Source: CAD feature listing. Evaluate the final solid. Frame: model axes, mm. Coordinates: 2 decimals unless noted, no trailing zeros. Order: outer loops, then holes, each group sorted by start corner. A loop starts at its lowest first (then second) coordinate and runs counter-clockwise, first axis right, second up.
```python
from build123d import *

# Parameters (mm, degrees)
EXTRUDE_1_DEPTH     = 2
SKETCH_2_R          = 3
SKETCH_2_R_2        = 0.8
CUT_EXTRUDE_1_DEPTH = 2
FILLET_1_R          = 2
FILLET_3_R          = 16


with BuildPart() as part:
    # Эскиз1 → Бобышка-Вытянуть1 (new body)
    with BuildSketch(Plane(origin=(0, 0, 0), x_dir=(0, 0, -1), z_dir=(1, 0, 0))):
        Polygon((-17.95, 0), (-3.95, 8), (3.95, 8), (17.95, 0), (17.95, -10), (-17.95, -10), align=None)
    extrude(amount=EXTRUDE_1_DEPTH)

    # Эскиз2 → Вырез-Вытянуть1 (cut)
    with BuildSketch(Plane(origin=(2, 0, 0), x_dir=(0, 0, -1), z_dir=(1, 0, 0))):
        with Locations((6.34428877, -4)):
            Circle(SKETCH_2_R)
        with Locations((1.84428877, -4)):
            Circle(SKETCH_2_R_2)
        with Locations((10.84428877, -4)):
            Circle(SKETCH_2_R_2)
    extrude(amount=-CUT_EXTRUDE_1_DEPTH, mode=Mode.SUBTRACT)

    # Скругление1
    fillet_1_edges = [part.edges().sort_by_distance(p)[0] for p in [
        (1, 0, 17.95),
        (1, 0, -17.95),
    ]]
    fillet(fillet_1_edges, radius=FILLET_1_R)

    # Скругление3
    # the kernel refuses this fillet: 16 mm, written as the material it takes off along each edge
    with BuildSketch(Plane(origin=(-10.622577483, 8, -3.95), x_dir=(0, 0, 1), z_dir=(1, 0, 0)), Plane(origin=(-10.622577483, 8, 3.95), x_dir=(0, -0.496138938356834, 0.868243142124459), z_dir=(1, 0, 0))) as fillet_3_piece_1:
        with BuildLine():
            CenterArc((FILLET_3_R * 0.265564437075, FILLET_3_R), FILLET_3_R, 240.255118703, 29.744881297)
            Line((-FILLET_3_R * 0.230574501282, FILLET_3_R * 0.131756857876), (0, 0))
            Line((0, 0), (FILLET_3_R * 0.265564437075, 0))
        make_face()
    extrude(amount=23.245154966, mode=Mode.SUBTRACT)


solid = part.part
```
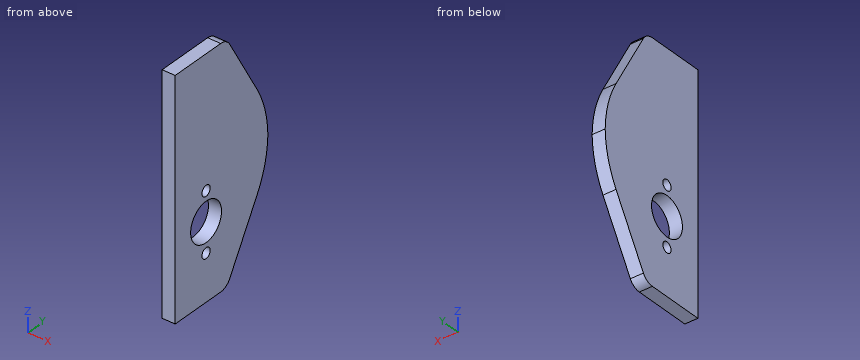
1. Section query C-C, the plane y = -1.5. Output: boundary loops of the cut face in (x, z), plus the area to 3 significant figures.
2. Material intervals for line 1 along Y through (x, z) = (1.4, -6); line 2 along Z through (x, y) = (1.15, -5.25); line 3 along Z through (x, y) = (0.4, -6.5), sorted ascending.
3. Section query A-A, the plane y = -4. Output: boundary loops of the cut face in (x, z).
4. Contact query for flat-ended pins moving along their axis: P1, Ø1, axis at x = 1, z = 10.5, coming from the +Y side; P2, Ø5.5, axis at y = -4, z = -6.34, coming from the -X side. Output: stop coordinate, or through.
5. Section query B-B, the plane x = 0.85. Output: boundary loops of the cut face in (y, z), plus the area to 3 significant figures.
6. Section query D-D, the plane z = -14. Output: boundary loops of the cut face in (x, y), plus the area to 3 significant figures.
Answer key:
1. outline: (0, -17.95) - (2, -17.95) - (2, -8) - (0, -8) - close; (0, -4.69) - (2, -4.69) - (2, 17.95) - (0, 17.95) - close
1. area: 65.2 mm2
2. line 1: y = -10 to -6.98, -1.02 to 6.71
2. line 2: z = -17.95 to -9.07, -3.62 to 17.95
2. line 3: z = -17.95 to -8, -4.69 to 17.95
3. outline: (0, -17.95) - (2, -17.95) - (2, -11.64) - (0, -11.64) - close; (0, -10.04) - (2, -10.04) - (2, -9.34) - (0, -9.34) - close; (0, -3.34) - (2, -3.34) - (2, -2.64) - (0, -2.64) - close; (0, -1.04) - (2, -1.04) - (2, 17.95) - (0, 17.95) - close
4. P1: stops at y = 4.54
4. P2: passes through
5. outline: (-10, -17.95) - (-1.16, -17.95) arc R2 ccw to (0.58, -16.94) - (5.89, -7.64) arc R16 ccw to (8, 0) arc R16 ccw to (5.89, 7.64) - (0.58, 16.94) arc R2 ccw to (-1.16, 17.95) - (-10, 17.95) - close; hole circle Ø6 at (-4, -6.34); hole circle Ø1.6 at (-4, -10.84); hole circle Ø1.6 at (-4, -1.84)
5. area: 498 mm2
6. outline: (0, -10) - (2, -10) - (2, 2.26) - (0, 2.26) - close
6. area: 24.5 mm2
